Work out the finished part from the listing and answer in its coordinate system (mm). A direction names the side the tool comes from. Coordinates: 2 decimals unless noted, no trailing zeros. Order: outer loops, then holes, each group sorted by start corner. A loop starts at its lowest first (then second) coordinate and runs counter-clockwise, first axis right, second up.
1. The part is cut by section B-B, the plane x = 13.5. Give the vertices of the cut face in (y, z) (3 decimals).
2. The part is cut by section A-A, the plane y = 0. Give the vertices of the cut face in (x, z).
3. Flat-ended cylindrical pins translate along their axes: pin 1 Ø4 at (x, z) = (50, 51.5) entering from +Y; pin 2 Ø1.5 at (y, z) = (44.5, 51) entering from -X; pin 3 Ø1.8 at (x, y) = (25.34, -110.21) entering from -Z; pin 4 Ø2 at (x, z) = (21, 49) entering from +Y. Find the tip coordinate at first contact, or state that the pin passes through.
4. Determine the mould class of faces 1 (the flat face through (32, -32, 53.75)), 2 (the flat face through (43.82, -27.96, 49.95)) for opening direction Y: +Y half, -Y half, draft (parallel to the pull), parting line (faces both ways), or undercut.
5. The part is cut by section C-C, the plane z = 51.5. Count the separate pieces of the cut face and the enclosed holes in it, then the cut area to 3 significant figures.
6. Find the intervals of material crossed by probe 1 along Y at (x, z) = (10, 49.75) (3 decimals); probe 2 along X at (y, z) = (4, 48); probe 3 along Y at (x, z) = (1.5, 50) (3 decimals), in increasing order.
7. A tool of negligible diameter and unlimited length cuts with its end or side. For faces 3 (the flat face through (32, -41, 46.25)), 4 (the flat face through (-19, 48.375, 50)), from which of +Z, -Z, +X, -X, +Y, -Y can it reach the whole face along a straight path? Write none if from no direction.
8. The part is cut by section D-D, the plane y = 28. Give the vertices of the cut face in (x, z), then the cut area to 3 significant figures.
```python
from build123d import *

# Parameters (mm, degrees)
SKETCH1_R           = 1000
SKETCH1_R_2         = 600
BOSS_EXTRUDE1_DEPTH = 100
ECHELLE1_SCALE      = 0.075
ESQUISSE1_R         = 1.5
BOSS_EXTRU_1_DEPTH  = 3
CONG_1_R            = 1
CONG_3_R            = 1
CHANFREIN1_SIZE     = 0.5


with BuildPart() as part:
    # Sketch1 → Boss-Extrude1 (new body)
    with BuildSketch(Plane.XY):
        Circle(SKETCH1_R)
        Circle(SKETCH1_R_2, mode=Mode.SUBTRACT)
        with BuildLine():
            Line((0, 615), (-500, 615))
            ThreePointArc((-500, 615), (-515, 630), (-500, 645))
            Line((-500, 645), (0, 645))
            ThreePointArc((0, 645), (15, 630), (0, 615))
        make_face(mode=Mode.SUBTRACT)
        with BuildLine():
            Line((361.48793016, 497.54545154), (-43.020567028, 791.438077687))
            ThreePointArc((-43.020567028, 791.438077687), (-46.339043159, 812.390111387), (-25.387009459, 815.708587518))
            Line((-25.387009459, 815.708587518), (379.121487729, 521.815961372))
            ThreePointArc((379.121487729, 521.815961372), (382.43996386, 500.863927672), (361.48793016, 497.54545154))
        make_face(mode=Mode.SUBTRACT)
        with BuildLine():
            Line((584.899757522, 190.04545154), (430.391260334, 665.573709688))
            ThreePointArc((430.391260334, 665.573709688), (440.021853163, 684.474812348), (458.922955823, 674.84421952))
            Line((458.922955823, 674.84421952), (613.43145301, 199.315961372))
            ThreePointArc((613.43145301, 199.315961372), (603.800860182, 180.414858712), (584.899757522, 190.04545154))
        make_face(mode=Mode.SUBTRACT)
        with BuildLine():
            Line((584.899757521, -190.045451541), (739.408254709, 285.482806607))
            ThreePointArc((739.408254709, 285.482806607), (758.309357369, 295.113399436), (767.939950198, 276.212296776))
            Line((767.939950198, 276.212296776), (613.43145301, -199.315961372))
            ThreePointArc((613.43145301, -199.315961372), (594.53035035, -208.946554201), (584.899757521, -190.045451541))
        make_face(mode=Mode.SUBTRACT)
        with BuildLine():
            Line((361.48793016, -497.545451541), (765.996427348, -203.652825394))
            ThreePointArc((765.996427348, -203.652825394), (786.948461048, -206.971301525), (783.629984916, -227.923335225))
            Line((783.629984916, -227.923335225), (379.121487729, -521.815961372))
            ThreePointArc((379.121487729, -521.815961372), (358.169454029, -518.497485241), (361.48793016, -497.545451541))
        make_face(mode=Mode.SUBTRACT)
        with BuildLine():
            Line((0, -615), (500, -615))
            ThreePointArc((500, -615), (515, -630), (500, -645))
            Line((500, -645), (0, -645))
            ThreePointArc((0, -645), (-15, -630), (0, -615))
        make_face(mode=Mode.SUBTRACT)
        with BuildLine():
            Line((-361.48793016, -497.54545154), (43.020567028, -791.438077687))
            ThreePointArc((43.020567028, -791.438077687), (46.339043159, -812.390111387), (25.387009459, -815.708587518))
            Line((25.387009459, -815.708587518), (-379.121487729, -521.815961372))
            ThreePointArc((-379.121487729, -521.815961372), (-382.43996386, -500.863927672), (-361.48793016, -497.54545154))
        make_face(mode=Mode.SUBTRACT)
        with BuildLine():
            Line((-584.899757522, -190.04545154), (-430.391260334, -665.573709688))
            ThreePointArc((-430.391260334, -665.573709688), (-440.021853163, -684.474812348), (-458.922955823, -674.84421952))
            Line((-458.922955823, -674.84421952), (-613.43145301, -199.315961372))
            ThreePointArc((-613.43145301, -199.315961372), (-603.800860182, -180.414858712), (-584.899757522, -190.04545154))
        make_face(mode=Mode.SUBTRACT)
        with BuildLine():
            Line((-584.899757521, 190.045451541), (-739.408254709, -285.482806607))
            ThreePointArc((-739.408254709, -285.482806607), (-758.309357369, -295.113399436), (-767.939950198, -276.212296776))
            Line((-767.939950198, -276.212296776), (-613.43145301, 199.315961372))
            ThreePointArc((-613.43145301, 199.315961372), (-594.53035035, 208.946554201), (-584.899757521, 190.045451541))
        make_face(mode=Mode.SUBTRACT)
        with BuildLine():
            Line((-361.48793016, 497.545451541), (-765.996427347, 203.652825394))
            ThreePointArc((-765.996427347, 203.652825394), (-786.948461048, 206.971301525), (-783.629984916, 227.923335225))
            Line((-783.629984916, 227.923335225), (-379.121487728, 521.815961372))
            ThreePointArc((-379.121487728, 521.815961372), (-358.169454028, 518.497485241), (-361.48793016, 497.545451541))
        make_face(mode=Mode.SUBTRACT)
    extrude(amount=BOSS_EXTRUDE1_DEPTH)


with BuildPart() as part_1:
    # Echelle1: scaled about (0, 0, 50)
    add(part.part.scale(ECHELLE1_SCALE).moved(Location((0, 0, 46.25))))

    # Esquisse1 → Boss.-Extru.1 (add)
    with BuildSketch(Plane(origin=(0, 0, 46.25), x_dir=(-1, 0, 0), z_dir=(0, 0, -1))):
        with BuildLine():
            Line((0.012013665, -104.11489824), (0.012013665, -116.31489824))
            Line((0.012013665, -116.31489824), (4.812013665, -116.31489824))
            Line((4.812013665, -116.31489824), (4.812013665, -74.845470968))
            ThreePointArc((4.812013665, -74.845470968), (-10.438835143, -74.26998533), (-25.257433458, -70.619133775))
            ThreePointArc((-25.257433458, -70.619133775), (-26.896134951, -72.45605199), (-27.487986335, -74.845470968))
            Line((-27.487986335, -74.845470968), (-27.487986335, -116.31489824))
            Line((-27.487986335, -116.31489824), (-22.687986335, -116.31489824))
            Line((-22.687986335, -116.31489824), (-22.687986335, -104.11489824))
            Line((-22.687986335, -104.11489824), (0.012013665, -104.11489824))
        make_face()
        with Locations((-25.337986335, -110.21489824)):
            Circle(ESQUISSE1_R, mode=Mode.SUBTRACT)
        with Locations((2.662013665, -110.21489824)):
            Circle(ESQUISSE1_R, mode=Mode.SUBTRACT)
    extrude(amount=-BOSS_EXTRU_1_DEPTH)

    # Congé1
    cong_1_edges = [part_1.edges().sort_by_distance(p)[0] for p in [
        (25.257433458, -70.619133775, 47.75),
    ]]
    fillet(cong_1_edges, radius=CONG_1_R)

    # Congé3
    cong_3_edges = [part_1.edges().sort_by_distance(p)[0] for p in [
        (-4.812013665, -74.845470968, 47.75),
    ]]
    fillet(cong_3_edges, radius=CONG_3_R)

    # Chanfrein1
    chanfrein1_edges = [part_1.edges().sort_by_distance(p)[0] for p in [
        (22.687986335, -110.21489824, 46.25),
        (11.337986335, -104.11489824, 46.25),
        (-0.012013665, -110.21489824, 46.25),
    ]]
    chamfer(chanfrein1_edges, length=CHANFREIN1_SIZE)


solid = part_1.part
```
Geometry says:
1. outline: (-104.115, 46.75) - (-103.615, 46.25) - (-48.375, 46.25) - (-48.375, 53.75) - (-73.775, 53.75) - (-73.775, 49.25) - (-104.115, 49.25) - close; (-46.125, 46.25) - (-42.927, 46.25) - (-42.927, 53.75) - (-46.125, 53.75) - close; (42.927, 46.25) - (47.205, 46.25) - (47.205, 53.75) - (42.927, 53.75) - close; (49.986, 46.25) - (73.775, 46.25) - (73.775, 53.75) - (49.986, 53.75) - close
2. outline: (-75, 46.25) - (-50.86, 46.25) - (-50.86, 53.75) - (-75, 53.75) - close; (-48.5, 46.25) - (-45, 46.25) - (-45, 53.75) - (-48.5, 53.75) - close; (45, 46.25) - (48.5, 46.25) - (48.5, 53.75) - (45, 53.75) - close; (50.86, 46.25) - (75, 46.25) - (75, 53.75) - (50.86, 53.75) - close
3. pin 1: stops at y = 57.63
3. pin 2: stops at x = -60.92
3. pin 3: passes through
3. pin 4: stops at y = 72.28
4. face 1: draft
4. face 2: undercut
5. separate pieces: 1
5. enclosed holes: 11
5. area: 10,400 mm2
6. probe 1: y = -74.33 to -48.375, -46.125 to -43.875, 43.875 to 49.748, 52.529 to 74.33
6. probe 2: x = -74.89 to -49.56, -47.2 to -44.82, 44.82 to 49.8, 52.16 to 74.89
6. probe 3: y = -74.985 to -60.885, -58.103 to -48.375, -46.125 to -44.975, 44.975 to 55.924, 58.705 to 74.985
7. face 3: -Z, +X, -X, +Y, -Y
7. face 4: +Z, -Z
8. outline: (-69.58, 46.25) - (-43.76, 46.25) - (-43.76, 53.75) - (-69.58, 53.75) - close; (-39.93, 46.25) - (-35.23, 46.25) - (-35.23, 53.75) - (-39.93, 53.75) - close; (35.23, 46.25) - (39.4, 46.25) - (39.4, 53.75) - (35.23, 53.75) - close; (41.77, 46.25) - (69.58, 46.25) - (69.58, 53.75) - (41.77, 53.75) - close
8. area: 469 mm2
